Design review of the part built by this model. Coordinates are the model's own, in mm. A direction names the side the tool comes from. Coordinates: 2 decimals unless noted, no trailing zeros. Loops run counter-clockwise (first coordinate to the right, second up) from the corner with the lowest first, then second, coordinate; pieces in that order, holes last.
Q1. Wall thickness on probe 1 along X at (y, z) = (-3, 16.5); probe 2 along Y at (x, z) = (-9.95, 25); probe 3 along Z at (x, y) = (-3.25, 15.5): over which ranges is each line inside the solid? List them lowest first.
Q2. Machinability: for faces 4 (the face through (-10, -12, 25)), 5 (the face through (12.5, 0, 14)), 6 (the face through (0, 12, 2)), 7 (the face through (-7.5, 0, 14)), which of the approach directions +Z, -Z, +X, -X, +Y, -Y give a long, thin tool a straight path to every point of the face, cutting with its end or side? Answer none if there is none.
Q3. Add section A-A on x = -3.5. Give the boundary of the cut face in (y, z).
Q4. Add section D-D on z = 28. Give the boundary of the cut face in (x, y), and give its area (3 significant figures).
Q5. Add section B-B on z = 37. Give the boundary of the cut face in (x, y).
Q6. Draft analysis for pull direction X (two halves, no side actions). For faces 1 (the face through (-0.217, 12.924, 2.473)), 2 (the face through (-0.11, -16.07, 1.5)), 3 (the face through (-11, -0.18, 1.43)), state which applies: released by +X, released by -X, zero draft, split by the parting line, or undercut.
Q7. Add section C-C on y = -13.9. Give the boundary of the cut face in (x, z).
Q8. For P1, Ø3, axis at x = 0, y = 13.9, coming from the +Z side; P2, Ø6, axis at x = 0, y = 12, coming from the -Z side; P3, Ø2.5, axis at x = -10.5, y = 0.5, coming from the -Z side; P4, Ø1.5, axis at x = 10, z = 25, coming from the -Y side, all flat-tipped, find the tip position at first contact; note any pin that passes through.
```python
from build123d import *

# Parameters (mm, degrees)
SKETCH1_W               = 20
SKETCH1_H               = 35
SKETCH1_R               = 1
SKETCH1_W_2             = 14
SKETCH1_H_2             = 24
BOSS_EXTRUDE1_DEPTH     = 5
SKETCH2_W               = 40
SKETCH2_H               = 35
BOSS_EXTRUDE2_DEPTH     = 2.5
CUT_EXTRUDE3_DEPTH      = 49.023431781
CUT_EXTRUDE3_DEPTH_BACK = 49.023431781
SKETCH3_W               = 14
SKETCH3_H               = 24
SKETCH3_R               = 1
FILLET1_R               = 5


with BuildPart() as part:
    # Sketch1 → Boss-Extrude1 (new body)
    with BuildSketch(Plane.XY):
        Rectangle(SKETCH1_W, SKETCH1_H)
        with Locations((0, 13.9)):
            Circle(SKETCH1_R, mode=Mode.SUBTRACT)
        with Locations(Location((0, -13.9, 0), (0, 0, 180))):
            Circle(SKETCH1_R, mode=Mode.SUBTRACT)
        Rectangle(SKETCH1_W_2, SKETCH1_H_2, mode=Mode.SUBTRACT)
    extrude(amount=BOSS_EXTRUDE1_DEPTH)

    # Sketch2 → Boss-Extrude2 (add, symmetric)
    with BuildSketch(Plane.ZY.offset(10)):
        with Locations((20, 0)):
            Rectangle(SKETCH2_W, SKETCH2_H)
    boss_extrude2 = extrude(amount=BOSS_EXTRUDE2_DEPTH, both=True)

    # Mirror3: Boss-Extrude2 across plane
    add(boss_extrude2.mirror(Plane(origin=(0, 0, 0), x_dir=(0, 0, 1), z_dir=(1, 0, 0))))

    # Sketch3 → Cut-Extrude3 (cut, two sides: drawn at the far end of the back side and taken through both)
    with BuildSketch(Plane(origin=(-7.5, 0, 0), x_dir=(0, 0, -1), z_dir=(1, 0, 0)).offset(-CUT_EXTRUDE3_DEPTH_BACK)):
        with Locations((-25, 0)):
            Rectangle(SKETCH3_W, SKETCH3_H)
        with Locations((-25, -13.9)):
            Circle(SKETCH3_R)
        with Locations((-25, 13.9)):
            Circle(SKETCH3_R)
    extrude(amount=CUT_EXTRUDE3_DEPTH + CUT_EXTRUDE3_DEPTH_BACK, mode=Mode.SUBTRACT)

    # Fillet1
    # the kernel refuses this fillet: 5 mm, written as the material it takes off along each edge
    with BuildSketch(Plane(origin=(-7.5, -12.5, 5), x_dir=(0, 0, -1), z_dir=(0, -1, 0))) as fillet1_piece_1_section:
        Polygon((0, 0), (FILLET1_R, 0), (FILLET1_R, -FILLET1_R), (0, -FILLET1_R), align=None)
    fillet1_piece_1 = extrude(amount=FILLET1_R, mode=Mode.PRIVATE)
    fillet1_piece_1 = fillet1_piece_1 - Plane(origin=(-7.5, -12.5, 5), x_dir=(0.7071067811865475, 0, 0.7071067811865475), z_dir=(0, -1, 0)) * Sphere(FILLET1_R, mode=Mode.PRIVATE)
    add(fillet1_piece_1, mode=Mode.SUBTRACT)
    with BuildSketch(Plane(origin=(7.5, -12.5, 5), x_dir=(0, 0, -1), z_dir=(0, -1, 0))) as fillet1_piece_2_section:
        Polygon((0, 0), (FILLET1_R, 0), (FILLET1_R, FILLET1_R), (0, FILLET1_R), align=None)
    fillet1_piece_2 = extrude(amount=FILLET1_R, mode=Mode.PRIVATE)
    fillet1_piece_2 = fillet1_piece_2 - Plane(origin=(7.5, -12.5, 5), x_dir=(-0.7071067811865475, 0, 0.7071067811865475), z_dir=(0, -1, 0)) * Sphere(FILLET1_R, mode=Mode.PRIVATE)
    add(fillet1_piece_2, mode=Mode.SUBTRACT)
    with BuildSketch(Plane(origin=(-7.5, 12.5, 5), x_dir=(-1, 0, 0), z_dir=(0, 0, -1))) as fillet1_piece_3_section:
        Polygon((0, 0), (FILLET1_R, 0), (FILLET1_R, FILLET1_R), (0, FILLET1_R), align=None)
    fillet1_piece_3 = extrude(amount=FILLET1_R, mode=Mode.PRIVATE)
    fillet1_piece_3 = fillet1_piece_3 - Plane(origin=(-7.5, 12.5, 5), x_dir=(0.7071067811865475, -0.7071067811865475, 0), z_dir=(0, 0, -1)) * Sphere(FILLET1_R, mode=Mode.PRIVATE)
    add(fillet1_piece_3, mode=Mode.SUBTRACT)
    with BuildSketch(Plane(origin=(7.5, 12.5, 5), x_dir=(0, 0, -1), z_dir=(1, 0, 0))) as fillet1_piece_4_section:
        Polygon((0, 0), (FILLET1_R, 0), (FILLET1_R, FILLET1_R), (0, FILLET1_R), align=None)
    fillet1_piece_4 = extrude(amount=FILLET1_R, mode=Mode.PRIVATE)
    fillet1_piece_4 = fillet1_piece_4 - Plane(origin=(7.5, 12.5, 5), x_dir=(0, -0.7071067811865475, 0.7071067811865475), z_dir=(1, 0, 0)) * Sphere(FILLET1_R, mode=Mode.PRIVATE)
    add(fillet1_piece_4, mode=Mode.SUBTRACT)
    with BuildSketch(Plane(origin=(-7.5, -17.5, 0), x_dir=(0, 0, 1), z_dir=(1, 0, 0)), Plane(origin=(-7.5, 17.5, 0), x_dir=(0, -1, 0), z_dir=(1, 0, 0))) as fillet1_piece_5:
        with BuildLine():
            CenterArc((FILLET1_R, -FILLET1_R), FILLET1_R, 90, 90)
            Line((0, -FILLET1_R), (0, 0))
            Line((0, 0), (FILLET1_R, 0))
        make_face()
    extrude(amount=15, mode=Mode.SUBTRACT)
    with BuildSketch(Plane(origin=(-12.5, 17.5, 5), x_dir=(0, -1, 0), z_dir=(0, 0, 1)), Plane(origin=(12.5, -17.5, 52.5), x_dir=(-1, 0, 0), z_dir=(0, 0, -1))) as fillet1_piece_6:
        with BuildLine():
            CenterArc((FILLET1_R, FILLET1_R), FILLET1_R, 180, 90)
            Line((0, FILLET1_R), (0, 0))
            Line((0, 0), (FILLET1_R, 0))
        make_face()
    extrude(amount=47.5, mode=Mode.SUBTRACT)
    with BuildSketch(Plane(origin=(-12.5, -17.5, 52.5), x_dir=(1, 0, 0), z_dir=(0, 0, -1)), Plane(origin=(12.5, 17.5, 5), x_dir=(0, -1, 0), z_dir=(0, 0, 1))) as fillet1_piece_7:
        with BuildLine():
            CenterArc((FILLET1_R, -FILLET1_R), FILLET1_R, 90, 90)
            Line((0, -FILLET1_R), (0, 0))
            Line((0, 0), (FILLET1_R, 0))
        make_face()
    extrude(amount=47.5, mode=Mode.SUBTRACT)
    with BuildSketch(Plane(origin=(12.5, -12.5, 0), x_dir=(-1, 0, 0), z_dir=(0, 1, 0))) as fillet1_piece_8:
        with BuildLine():
            CenterArc((FILLET1_R, FILLET1_R), FILLET1_R, 180, 90)
            Line((0, FILLET1_R), (0, 0))
            Line((0, 0), (FILLET1_R, 0))
        make_face()
    extrude(amount=25, mode=Mode.SUBTRACT)
    with BuildSketch(Plane(origin=(-12.5, -12.5, 0), x_dir=(1, 0, 0), z_dir=(0, 1, 0))) as fillet1_piece_9:
        with BuildLine():
            CenterArc((FILLET1_R, -FILLET1_R), FILLET1_R, 90, 90)
            Line((0, -FILLET1_R), (0, 0))
            Line((0, 0), (FILLET1_R, 0))
        make_face()
    extrude(amount=25, mode=Mode.SUBTRACT)


solid = part.part
```
Entries:
1. probe 1: x = -12.5 to -7.5, 7.5 to 12.5
1. probe 2: y = -16.86 to -14.9, -12.9 to -12, 12 to 12.9, 14.9 to 16.86
1. probe 3: z = 1 to 5
2. face 4: +X, -X
2. face 5: +Z, -Z, +X, +Y, -Y
2. face 6: +Z, -Z
2. face 7: +Z, +Y, -Y
3. outline: (-17.5, 5) arc R5 ccw to (-12.5, 0) - (-12, 0) - (-12, 5) - close; (12, 0) - (12.5, 0) arc R5 ccw to (17.5, 5) - (12, 5) - close
4. outline: (-12.5, -12.5) arc R5 ccw to (-7.5, -17.5) - (-7.5, -12) - (-12.5, -12) - close; (-12.5, 12) - (-7.5, 12) - (-7.5, 17.5) arc R5 ccw to (-12.5, 12.5) - close; (7.5, -17.5) arc R5 ccw to (12.5, -12.5) - (12.5, -12) - (7.5, -12) - close; (7.5, 12) - (12.5, 12) - (12.5, 12.5) arc R5 ccw to (7.5, 17.5) - close
4. area: 88.5 mm2
5. outline: (-12.5, -12.5) arc R5 ccw to (-7.5, -17.5) - (-7.5, 17.5) arc R5 ccw to (-12.5, 12.5) - close; (7.5, -17.5) arc R5 ccw to (12.5, -12.5) - (12.5, 12.5) arc R5 ccw to (7.5, 17.5) - close
6. face 1: undercut
6. face 2: zero draft
6. face 3: released by -X
7. outline: (-12.3, 5) arc R4.8 ccw to (-7.5, 0.2) - (-1, 0.2) - (-1, 5) - (-7.5, 5) - (-7.5, 24) - (-12.3, 24) - close; (-12.3, 26) - (-7.5, 26) - (-7.5, 40) - (-12.3, 40) - close; (1, 0.2) - (7.5, 0.2) arc R4.8 ccw to (12.3, 5) - (12.3, 24) - (7.5, 24) - (7.5, 5) - (1, 5) - close; (7.5, 26) - (12.3, 26) - (12.3, 40) - (7.5, 40) - close
8. P1: stops at z = 5
8. P2: stops at z = 0
8. P3: stops at z = 0.32
8. P4: stops at y = -17.18
